```python
from build123d import *

# Parameters (mm, degrees)
SKETCH_1_W          = 200
SKETCH_1_H          = 120
SKETCH_1_R          = 15
EXTRUDE_1_DEPTH     = 10
SKETCH_2_W          = 200
SKETCH_2_H          = 45
EXTRUDE_2_DEPTH     = 100
SKETCH_3_R          = 5
CUT_EXTRUDE_1_DEPTH = 186.47236991


with BuildPart() as part:
    # 草图1 → 凸台-拉伸1 (new body)
    with BuildSketch(Plane.XY):
        Rectangle(SKETCH_1_W, SKETCH_1_H)
        Circle(SKETCH_1_R, mode=Mode.SUBTRACT)
    extrude(amount=EXTRUDE_1_DEPTH)

    # 草图2 → 凸台-拉伸2 (add)
    with BuildSketch(Plane(origin=(0, 0, 0), x_dir=(-1, 0, 0), z_dir=(0, 0, -1))):
        with Locations((0, 37.5)):
            Rectangle(SKETCH_2_W, SKETCH_2_H)
        with Locations((0, -37.5)):
            Rectangle(SKETCH_2_W, SKETCH_2_H)
    extrude(amount=EXTRUDE_2_DEPTH)

    # 草图3 → 切除-拉伸1 (cut, through all)
    with BuildSketch(Plane(origin=(0, 60, 0), x_dir=(1, 0, 0), z_dir=(0, 1, 0))):
        with Locations(Location((0, 80, 0), (0, 0, 180))):
            Circle(SKETCH_3_R)
        Polygon((-100, 5), (-100, 100), (-20, 100), (-40, 5), align=None)
        Polygon((100, 100), (20, 100), (40, 5), (100, 5), align=None)
    extrude(amount=-CUT_EXTRUDE_1_DEPTH, mode=Mode.SUBTRACT)


solid = part.part
```
Geometry: final body of the model. Coordinates: model frame, mm. A direction names the side the tool comes from. Coordinates: 2 decimals unless noted, no trailing zeros. Order: outer loops, then holes, each group sorted by start corner. A loop starts at its lowest first (then second) coordinate and runs counter-clockwise, first axis right, second up. Notation, with made-up numbers: (15.5, 71) -> (49.5, 71) arc R36 cw to (49.5, 107) -> close; hole circle Ø9 at (28.25, 29). An arc over 180 degrees is marked (long way). Use CSV: the item, a comma, the result in double quotes.
1) Section A-A on y = 0. Output: boundary loops of the cut face in (x, z), then the cut area to 3 significant figures.
Findings:
outline,"(-100, 0) -> (-15, 0) -> (-15, 10) -> (-100, 10) -> close; (15, 0) -> (100, 0) -> (100, 10) -> (15, 10) -> close"
area,"1,700 mm^2"
2) Line query: line 1 (Y direction, x = -16, z = -46.5); line 2 (Z direction, x = 0, y = -32); line 3 (X direction, y = -1, z = 0.5). Output: solid intervals per line, ascending.
Findings:
line 1,"y = -60 to -15, 15 to 60"
line 2,"z = -100 to -85, -75 to 10"
line 3,"x = -100 to -14.97, 14.97 to 100"
3) Mould query, pull axis X, two halves, no side actions, for faces 1 (the flat face through (-24, 1, 10)), 2 (the cylindrical face through (-14.985, 0.66, 4.93)), 3 (the flat face through (29.86, 37.82, -53.16)). Classes: +X half, -X half, draft (parallel to the pull), parting line (faces both ways), or undercut.
Findings:
face 1,"draft"
face 2,"undercut"
face 3,"+X half"
4) Section C-C on z = -80. Output: boundary loops of the cut face in (x, y), then the cut area to 3 significant figures.
Findings:
outline,"(-24.21, -60) -> (-5, -60) -> (-5, -15) -> (-24.21, -15) -> close; (-24.21, 15) -> (-5, 15) -> (-5, 60) -> (-24.21, 60) -> close; (5, -60) -> (24.21, -60) -> (24.21, -15) -> (5, -15) -> close; (5, 15) -> (24.21, 15) -> (24.21, 60) -> (5, 60) -> close"
area,"3,460 mm^2"
5) Section B-B on z = -67. Output: boundary loops of the cut face in (x, y).
Findings:
outline,"(-26.95, -60) -> (26.95, -60) -> (26.95, -15) -> (-26.95, -15) -> close; (-26.95, 15) -> (26.95, 15) -> (26.95, 60) -> (-26.95, 60) -> close"
6) Access query for faces 4 (the cylindrical face through (1.08, -37.18, -84.88)), 5 (the flat face through (70, 38, -5)), 6 (the flat face through (0, -37, -100)), 7 (the flat face through (-70, -37, -5)), 8 (the flat face through (-62, 0, 0)). Directions: +Z, -Z, +X, -X, +Y, -Y. A direction counts if a zero-diameter tool reaches every point of the face in a straight line with its end or side. Return the directions, or none.
Findings:
face 4,"+Y, -Y"
face 5,"-Z, +X, +Y, -Y"
face 6,"-Z, +X, -X, +Y, -Y"
face 7,"-Z, -X, +Y, -Y"
face 8,"-Z, +X, -X"
7) Section D-D on y = -18.5. Output: boundary loops of the cut face in (x, z).
Findings:
outline,"(-100, -5) -> (-40, -5) -> (-20, -100) -> (20, -100) -> (40, -5) -> (100, -5) -> (100, 10) -> (-100, 10) -> close; hole circle Ø10 at (0, -80)"
8) Pin query (flat end, axial travel): pin 1 Ø13.5 at (x, y) = (-73.5, -38) entering from -Z; pin 2 Ø24 at (x, y) = (-68, -2.5) entering from -Z. Return the tip coordinate at first contact, or that it passes through.
Findings:
pin 1,"stops at z = -5"
pin 2,"stops at z = 0"
